```python
from build123d import *

# Parameters (mm, degrees)
SKETCH1_W               = 1000
SKETCH1_H               = 550
BASE_EXTRUDE_DEPTH      = 150
SKETCH2_W               = 900
SKETCH2_H               = 450
CUT_EXTRUDE1_DEPTH      = 148
SHELL3_START            = -998
SHELL3_OUTLINE_W        = 546
SHELL3_OUTLINE_H        = 146
SHELL3_DEPTH            = 996
SKETCH3_W               = 50
SKETCH3_H               = 450
BOSS_EXTRUDE1_DEPTH     = 2
SKETCH4_R               = 2
BOSS_EXTRUDE2_DEPTH     = 10
MIRROR2_COPY_1_SKETCH_R = 2
MIRROR2_COPY_1_DEPTH    = 10


# Read off the part's stored shape, not the designer's step: Shell3
with BuildPart() as part:
    # Sketch1 → Base-Extrude (new body)
    with BuildSketch(Plane.XY):
        with Locations((-500, 275)):
            Rectangle(SKETCH1_W, SKETCH1_H)
    extrude(amount=BASE_EXTRUDE_DEPTH)

    # Sketch2 → Cut-Extrude1 (cut)
    with BuildSketch(Plane.XY.offset(150)):
        with Locations((-500, 275)):
            Rectangle(SKETCH2_W, SKETCH2_H)
    extrude(amount=-CUT_EXTRUDE1_DEPTH, mode=Mode.SUBTRACT)

    # Shell3 outline → Shell3 (cut)
    with BuildSketch(Plane.YZ.offset(SHELL3_START)):
        with Locations((275, 75)):
            Rectangle(SHELL3_OUTLINE_W, SHELL3_OUTLINE_H)
    extrude(amount=SHELL3_DEPTH, mode=Mode.SUBTRACT)

    # Sketch3 → Boss-Extrude1 (add)
    with BuildSketch(Plane.XY.offset(150)):
        with Locations((-500, 275)):
            Rectangle(SKETCH3_W, SKETCH3_H)
    extrude(amount=-BOSS_EXTRUDE1_DEPTH)

    # Sketch4 → Boss-Extrude2 (add)
    with BuildSketch(Plane.XZ.offset(-125)):
        with BuildLine():
            Line((-41, 150), (-33, 150))
            Line((-33, 150), (-33, 158))
            ThreePointArc((-33, 158), (-37, 162), (-41, 158))
            Line((-41, 158), (-41, 150))
        make_face()
        with Locations((-37, 158)):
            Circle(SKETCH4_R, mode=Mode.SUBTRACT)
    boss_extrude2 = extrude(amount=-BOSS_EXTRUDE2_DEPTH)

    # Mirror1: Boss-Extrude2 across plane
    add(boss_extrude2.mirror(Plane.ZY.offset(500)))

    # Mirror2: Boss-Extrude2 across plane
    add(boss_extrude2.mirror(Plane(origin=(0, 275, 0), x_dir=(0, 0, 1), z_dir=(0, -1, 0))))

    # Mirror2 copy 1 sketch → Mirror2 copy 1 (add)
    with BuildSketch(Plane(origin=(-1000, 425, 0), x_dir=(-1, 0, 0), z_dir=(0, 1, 0))):
        with BuildLine():
            Line((-41, 150), (-33, 150))
            Line((-33, 150), (-33, 158))
            ThreePointArc((-33, 158), (-37, 162), (-41, 158))
            Line((-41, 158), (-41, 150))
        make_face()
        with Locations((-37, 158)):
            Circle(MIRROR2_COPY_1_SKETCH_R, mode=Mode.SUBTRACT)
    extrude(amount=-MIRROR2_COPY_1_DEPTH)


solid = part.part
```
Geometry check sheet. Reference: the model listing, model coordinates, mm. A direction names the side the tool comes from. Coordinates: 2 decimals unless noted, no trailing zeros. Order: outer loops, then holes, each group sorted by start corner. A loop starts at its lowest first (then second) coordinate and runs counter-clockwise, first axis right, second up. Notation, with made-up numbers: (-33.75, 25) - (21.25, 25) arc R20 ccw to (21.25, 37) - close; hole circle Ø8 at (33, -6). An arc over 180 degrees is marked (long way). Answer in a Markdown table with one row per item. Add a question column.
1. Access from +Z, -Z, +X, -X, +Y, -Y to the whole of each face (thin tool, end or side, straight path). Record for faces 1 (the face through (-507, 550, 74)), 2 (the face through (-998, 271, 76)).
2. Material ranges on L1, parallel to X at y = 419.5, z = 158; L2, parallel to X at y = 361, z = 7; L3, parallel to Y at x = -330.5, z = 10, recorded low to high. Write a range as [from, to].
3. Section check B-B (y = 453.5). Enter the section's corners in (x, z).
4. Section check C-C (x = -613). Enter the section's corners in (y, z), plus the area to 3 significant figures.
5. Draft check along Y on faces 3 (the face through (-507, 0, 74)), 4 (the face through (-507, 279, 0)), 5 (the face through (-502, 274, 148)). Enter one of: +Y half, -Y half, draft (parallel to the pull), parting line (faces both ways), or undercut.
6. Section check A-A (z = 50). Enter the section's corners in (x, y).
7. Gauge pin test, flat ends, axial feed: pin 1 Ø10 at (x, z) = (-690.5, 59) entering from -Y; pin 2 Ø9 at (x, z) = (-38.5, 156) entering from -Y; pin 3 Ø4 at (y, z) = (131.5, 152.5) entering from +X; pin 4 Ø3 at (x, z) = (-963, 158) entering from +Y. Record the tip position at first contact, or that the pin passes through.
Data:
| question | item | result |
|---|---|---|
| 1 | face 1 | +Z, -Z, +X, -X, +Y |
| 1 | face 2 | none |
| 2 | L1 | x = [-967, -965], [-961, -959], [-41, -39], [-35, -33] |
| 2 | L2 | x = [-1000, -998], [-2, 0] |
| 2 | L3 | y = [0, 2], [548, 550] |
| 3 | outline | (-1000, 0) - (0, 0) - (0, 150) - (-50, 150) - (-50, 148) - (-2, 148) - (-2, 2) - (-998, 2) - (-998, 148) - (-950, 148) - (-950, 150) - (-1000, 150) - close; (-525, 148) - (-475, 148) - (-475, 150) - (-525, 150) - close |
| 4 | outline | (0, 0) - (550, 0) - (550, 150) - (500, 150) - (500, 148) - (548, 148) - (548, 2) - (2, 2) - (2, 148) - (50, 148) - (50, 150) - (0, 150) - close |
| 4 | area | 1,880 mm² |
| 5 | face 3 | -Y half |
| 5 | face 4 | draft |
| 5 | face 5 | undercut |
| 6 | outline | (-1000, 0) - (0, 0) - (0, 550) - (-1000, 550) - close; hole (-998, 2) - (-2, 2) - (-2, 548) - (-998, 548) - close |
| 7 | pin 1 | stops at y = 0 |
| 7 | pin 2 | stops at y = 125 |
| 7 | pin 3 | stops at x = -33 |
| 7 | pin 4 | passes through |
